For this review, take the finished solid that the model builds, in its own axes (mm). Face numbers are marked on the shaded views. Give positions to 0.01 mm unless a question says otherwise; leave off trailing zeros. Write each loop counter-clockwise with the first axis right and the second up, starting at its lowest first coordinate (ties: lowest second). Pieces come first, ordered by that corner, then holes.
Q1. We need section B-B (x = -7.5). Write out the cut boundary in (y, z).
Q2. We need section A-A (z = 2.8). Write out the cut boundary in (x, y).
Q3. We need section D-D (z = 2). Write out the cut boundary in (x, y).
Q4. We need section C-C (y = -0.9). Write out the cut boundary in (x, z), then the cut area to 3 significant figures.
Q5. Mouldability with a two-part tool opening along X and no side actions: class the marked faces 1, 2 and 3 as released by +X, released by -X, zero draft, split by the parting line, or undercut.
Q6. For line 1 (Z direction, x = 7.5, y = -1.5); line 2 (X direction, y = 0.4, z = 1.3); line 3 (X direction, y = -2.6, z = 1.2), list the stretches that pass through material, from the lowest coordinate up.
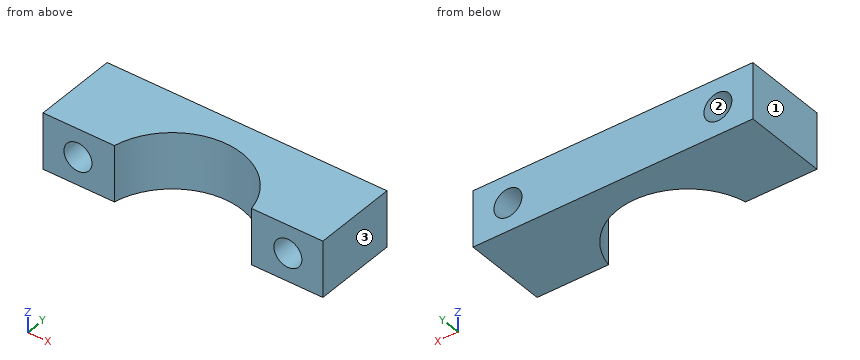
```python
from build123d import *

# Parameters (mm, degrees)
EXTRUDE1_DEPTH = 4
SKETCH2_R      = 1
EXTRUDE2_DEPTH = 7


with BuildPart() as part:
    # Sketch1 → Extrude1 (new body)
    with BuildSketch(Plane.XY):
        with BuildLine():
            Line((4.898979486, -3), (10, -3))
            Line((10, -3), (10, 3))
            Line((10, 3), (-10, 3))
            Line((-10, 3), (-10, -3))
            Line((-10, -3), (-4.898979486, -3))
            ThreePointArc((-4.898979486, -3), (0, 1), (4.898979486, -3))
        make_face()
    extrude(amount=EXTRUDE1_DEPTH)

    # Sketch2 → Extrude2 (cut, through all)
    with BuildSketch(Plane.XZ.offset(3)):
        with Locations((-7.5, 2)):
            Circle(SKETCH2_R)
    extrude2 = extrude(amount=-EXTRUDE2_DEPTH, mode=Mode.SUBTRACT)

    # Mirror1: Extrude2 across plane
    add(extrude2.mirror(Plane(origin=(0, 0, 0), x_dir=(0, 0, 1), z_dir=(1, 0, 0))), mode=Mode.SUBTRACT)


solid = part.part
```
Computed:
1. outline: (-3, 0) - (3, 0) - (3, 1) - (-3, 1) - close; (-3, 3) - (3, 3) - (3, 4) - (-3, 4) - close
2. outline: (-10, -3) - (-8.1, -3) - (-8.1, 3) - (-10, 3) - close; (-6.9, -3) - (-4.9, -3) arc R5 cw to (4.9, -3) - (6.9, -3) - (6.9, 3) - (-6.9, 3) - close; (8.1, -3) - (10, -3) - (10, 3) - (8.1, 3) - close
3. outline: (-10, -3) - (-8.5, -3) - (-8.5, 3) - (-10, 3) - close; (-6.5, -3) - (-4.9, -3) arc R5 cw to (4.9, -3) - (6.5, -3) - (6.5, 3) - (-6.5, 3) - close; (8.5, -3) - (10, -3) - (10, 3) - (8.5, 3) - close
4. outline: (-10, 0) - (-3.92, 0) - (-3.92, 4) - (-10, 4) - close; (3.92, 0) - (10, 0) - (10, 4) - (3.92, 4) - close; hole circle Ø2 at (-7.5, 2); hole circle Ø2 at (7.5, 2)
4. area: 42.3 mm2
5. face 1: released by -X
5. face 2: undercut
5. face 3: released by +X
6. line 1: z = 0 to 1, 3 to 4
6. line 2: x = -10 to -8.21, -6.79 to -2.37, 2.37 to 6.79, 8.21 to 10
6. line 3: x = -10 to -8.1, -6.9 to -4.8, 4.8 to 6.9, 8.1 to 10
